from build123d import *

# Parameters (mm, degrees)
M8_SHCS_IN_HAV_A1_D               = 9
M8_SHCS_IN_HAV_A1_CBORE_D         = 15
M8_SHCS_IN_HAV_A1_CBORE_DEPTH     = 8
M12X1_75_DI_LI_DELIK1_D           = 10.2
M12X1_75_DI_LI_DELIK1_CSINK_D     = 12.05
M12X1_75_DI_LI_DELIK1_CSINK_ANGLE = 90


with BuildPart() as part:
    # Çizim1 → Döndür1 (revolve)
    with BuildSketch(Plane.XY, mode=Mode.PRIVATE) as d_nd_r1_sk:
        Polygon((-47.583548513, 30), (-7.583548513, 30), (-7.583548513, 50), (-27.583548513, 50), (-27.583548513, 150), (-47.583548513, 150), align=None)
    revolve(d_nd_r1_sk.sketch.rotate(Axis((-58.347943389, 0, 0), (1, 0, 0)), 90), axis=Axis((-58.347943389, 0, 0), (1, 0, 0)))

    # M8 SHCS İçin Havşa1 (through all)
    with Locations(Plane(origin=(-27.583548513, 0, 0), x_dir=(0, 0, -1), z_dir=(1, 0, 0))):
        with Locations((80, 0), (401.288725226, 148.981360789), (40, -69.282032303), (-40, -69.282032303), (-80, 0), (-40, 69.282032303), (40, 69.282032303), (0, 0)):
            CounterBoreHole(M8_SHCS_IN_HAV_A1_D / 2, M8_SHCS_IN_HAV_A1_CBORE_D / 2, M8_SHCS_IN_HAV_A1_CBORE_DEPTH)

    # M12x1.75 Dişli Delik1 (through all)
    with Locations(Plane(origin=(-27.583548513, 0, 0), x_dir=(0, 0, -1), z_dir=(1, 0, 0))):
        with Locations((110, 0), (95.262794416, -55), (55, -95.262794416), (0, -110), (-55, -95.262794416), (-95.262794416, -55), (-110, 0), (-95.262794416, 55), (-55, 95.262794416), (0, 110), (55, 95.262794416), (95.262794416, 55), (0, 0)):
            CounterSinkHole(M12X1_75_DI_LI_DELIK1_D / 2, M12X1_75_DI_LI_DELIK1_CSINK_D / 2, counter_sink_angle=M12X1_75_DI_LI_DELIK1_CSINK_ANGLE)


solid = part.part
Input: part model. Units: mm. Frame: model coordinates. A direction names the side the tool comes from. Give positions to 0.01 mm unless a question says otherwise; leave off trailing zeros. Write each loop counter-clockwise with the first axis right and the second up, starting at its lowest first coordinate (ties: lowest second). Pieces come first, ordered by that corner, then holes. Notation, with made-up numbers: M 55,67.25 L 86,67.25 A33 cw 86,104.25 Z; hole C 23.25,-11.5 d8. An arc over 180 degrees is marked long. Write item = value, one per line. Start each with the question number.
1) Reachability of faces 1 (the flat face through (-35.584, -5, -80)), 2 (the cylindrical face through (-38.18, 0.224, 104.905)) from +Z, -Z, +X, -X, +Y, -Y: full face, straight path, thin tool, end or side. Return the list, or none.
2) Material intervals for line 1 along Y through (x, z) = (-37, 0); line 2 along Z through (x, y) = (-41.5, -99.5); line 3 along Y through (x, z) = (-35, 55), sorted ascending. Write a range as [from, to].
3) First-contact query: pin 1 Ø3 at (x, y) = (-33.5, 1) entering from -Z; pin 2 Ø1 at (y, z) = (79, 114.5) entering from +X; pin 3 Ø4.5 at (y, z) = (-2, -77.5) entering from +X; pin 4 Ø6 at (x, y) = (-21.5, 21.5) entering from -Z. Flat tips, straight axial feed; report the tip coordinate or a pass-through.
4) Cut plane B-B on x = -14. Return the cut outline in (y, z).
5) Draft query along Y for faces 3 (the cylindrical face through (-31.528, 76.718, -39.024)), 4 (the flat face through (-7.584, 22, -22)). Return one class per face: +Y half, -Y half, draft (parallel to the pull), parting line (faces both ways), or undercut.
6) Cut plane C-C on z = 55. Return the cut outline in (x, y).
7) Cut plane A-A on x = -39. Count the separate pieces of the cut face and the enclosed holes in it, then the cut area to 3 significant figures.
8) Cut plane D-D on y = 129. Return the cut outline in (x, z), then the cut area to 3 significant figures.
Solved:
q1.face_1 = +X
q1.face_2 = +X, -X
q2.line_1 = [-150, -115.1], [-104.9, -30], [30, 104.9], [115.1, 150]
q2.line_2 = [-112.25, -57.84], [-52.16, 52.16], [57.84, 112.25]
q2.line_3 = [-139.55, -100.36], [-90.16, 90.16], [100.36, 139.55]
q3.pin_1 = -150
q3.pin_2 = -27.58
q3.pin_3 = -35.58
q3.pin_4 = -46.45
q4.outline = C 0,0 d100; hole C 0,0 d60
q5.face_3 = undercut
q5.face_4 = draft
q6.outline = M -47.58,-139.55 L -27.58,-139.55 L -27.58,-101.29 L -28.51,-100.36 L -47.58,-100.36 Z; M -47.58,-90.16 L -28.51,-90.16 L -27.58,-89.24 L -27.58,89.24 L -28.51,90.16 L -47.58,90.16 Z; M -47.58,100.36 L -28.51,100.36 L -27.58,101.29 L -27.58,139.55 L -47.58,139.55 Z
q7.separate_pieces = 1
q7.enclosed_holes = 19
q7.area = 66,500 mm2
q8.outline = M -47.58,-76.54 L -27.58,-76.54 L -27.58,76.54 L -47.58,76.54 Z
q8.area = 3,060 mm2
